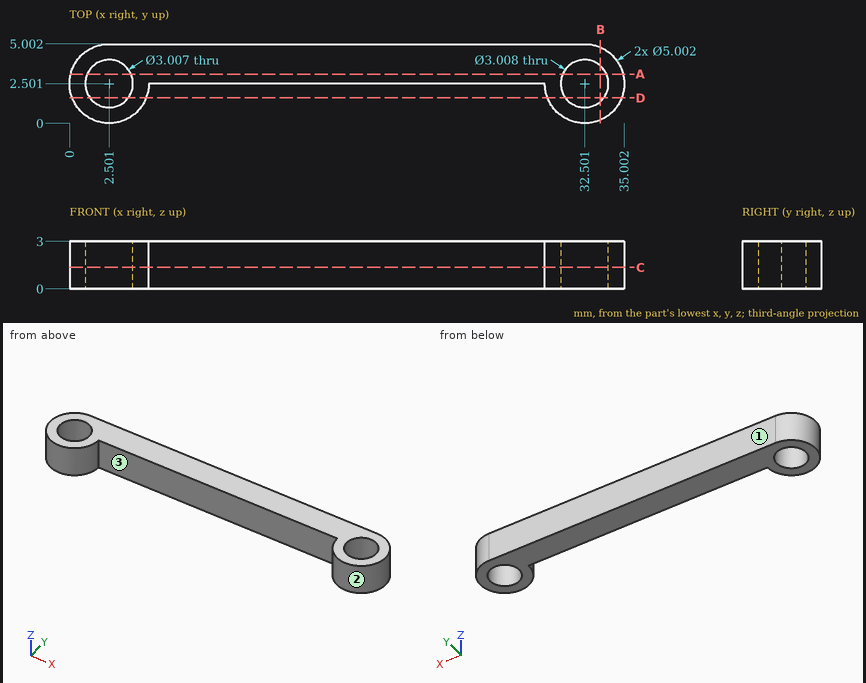
Geometry check sheet. Reference: drawing and pictorial views, mm from the part's lowest x, y, z. Give positions to 0.01 mm unless a question says otherwise; leave off trailing zeros. Write each loop counter-clockwise with the first axis right and the second up, starting at its lowest first coordinate (ties: lowest second). Pieces come first, ordered by that corner, then holes.
Item 1: Cross-section at C-C (z = 1.35). Enter the section's corners in (x, y) (1 decimal).
Item 2: Gauge pin test, flat ends, axial feed: pin 1 (1.5 mm diameter, centred on x = 12.5, z = 2, fed in from -Y); pin 2 (1.5 mm diameter, centred on y = 1, z = 1, fed in from -X) (1 decimal). Record the tip position at first contact, or that the pin passes through.
Item 3: Cross-section at B-B (x = 33.5). Enter the section's corners in (y, z) (1 decimal).
Item 4: Scan lines: L1, parallel to X at y = 2.55, z = 2.4 (1 decimal); L2, parallel to X at y = 2.45, z = 2.75 (1 decimal); L3, parallel to X at y = 3.4, z = 1.5 (1 decimal). Record each from-to range of solid material in increasing order.
Item 5: Cross-section at A-A (y = 3.1). Enter the section's corners in (x, z).
Item 6: Draft check along X on the marked faces 1, 2 and 3. Enter one of: released by +X, released by -X, zero draft, split by the parting line, or undercut.
Item 7: Cross-section at D-D (y = 1.6). Enter the section's corners in (x, z) (1 decimal).
Report:
1. outline: (2.5, 5) arc R2.5 ccw (long way) to (5, 2.5) - (30, 2.5) arc R2.5 ccw (long way) to (32.5, 5) - close; hole circle Ø3 at (2.5, 2.5); hole circle Ø3 at (32.5, 2.5)
2. pin 1: stops at y = 2.5
2. pin 2: stops at x = 0.1
3. outline: (0.2, 0) - (1.4, 0) - (1.4, 3) - (0.2, 3) - close; (3.6, 0) - (4.8, 0) - (4.8, 3) - (3.6, 3) - close
4. L1: x = 0 to 1, 4 to 31, 34 to 35
4. L2: x = 0 to 1, 4 to 5, 30 to 31, 34 to 35
4. L3: x = 0.2 to 1.3, 3.7 to 31.3, 33.7 to 34.8
5. outline: (0.07, 0) - (1.12, 0) - (1.12, 3) - (0.07, 3) - close; (3.88, 0) - (31.12, 0) - (31.12, 3) - (3.88, 3) - close; (33.88, 0) - (34.93, 0) - (34.93, 3) - (33.88, 3) - close
6. face 1: zero draft
6. face 2: undercut
6. face 3: undercut
7. outline: (0.2, 0) - (1.3, 0) - (1.3, 3) - (0.2, 3) - close; (3.7, 0) - (4.8, 0) - (4.8, 3) - (3.7, 3) - close; (30.2, 0) - (31.3, 0) - (31.3, 3) - (30.2, 3) - close; (33.7, 0) - (34.8, 0) - (34.8, 3) - (33.7, 3) - close
